```python
from build123d import *

# Parameters (mm, degrees)
F0_W     = 50
F0_H     = 7
F1_DEPTH = 25
F2_SIZE  = 2.4
F3_R     = 0.6
F4_DEPTH = 16.5
F5_R     = 0.59999


# Not quite as in the source:
# - a fillet or chamfer is up to 0.001 mm smaller than in the source, because OpenCascade refuses the exact size


with BuildPart() as f1:
    # F0 (on Top) → F1 (new body)
    with BuildSketch(Plane.XY):
        Rectangle(F0_W, F0_H)
    extrude(amount=F1_DEPTH)

    # F2
    f2_edges = [f1.edges().sort_by_distance(p)[0] for p in [
        (0, -3.5, 25),
        (0, 3.5, 25),
    ]]
    chamfer(f2_edges, length=F2_SIZE)

    # F3 (on Right) → F4 (join, symmetric)
    with BuildSketch(Plane.YZ):
        with Locations((0, 25)):
            Circle(F3_R)
    extrude(amount=F4_DEPTH, both=True)

    # F5 (radius 0.6 in the source; OpenCascade refuses exactly that, so slightly less here)
    f5_edges = [f1.edges().sort_by_distance(p)[0] for p in [
        (16.5, 0, 25.6),
        (-16.5, 0, 25.6),
    ]]
    fillet(f5_edges, radius=F5_R)


solid = f1.part
```
CAD build for the part. Positions are in the model's coordinates, mm. A direction names the side the tool comes from. Round coordinates to 2 decimals unless told otherwise and drop trailing zeros. Order: outer loops, then holes, each group sorted by start corner. A loop starts at its lowest first (then second) coordinate and runs counter-clockwise, first axis right, second up.
Item 1: Saw through at B-B on y = 2.5. Write the cut outline in (x, z).
Item 2: Pin check, flat tips, straight feed: pin 1 (0.7 mm diameter, centred on x = -5.5, y = 0.5, fed in from +Z); pin 2 (3 mm diameter, centred on x = -19.5, y = 2.5, fed in from +Z). Stop position of each tip, or through.
Item 3: Tool access for faces 1 (the face through (0.2, 0, 25.6)), 2 (the face through (-0.35, 0.75, 25)): list every direction of +Z, -Z, +X, -X, +Y, -Y with a clear straight run to the whole face (end or side of a thin tool).
Item 4: Saw through at A-A on x = -21. Write the cut outline in (y, z).
Item 5: Probe line 1 along Z through (x, y) = (-18.5, 1); line 2 along Z through (x, y) = (-16, 0); line 3 along Y through (x, z) = (-4, 23). List the from-to ranges inside material, lowest first.
Item 6: Saw through at C-C on x = 9.5. Write the cut outline in (y, z).
Reported:
1. outline: (-25, 0) - (25, 0) - (25, 23.6) - (-25, 23.6) - close
2. pin 1: stops at z = 25.58
2. pin 2: stops at z = 25
3. face 1: +Z, +X, -X
3. face 2: +Z
4. outline: (-3.5, 0) - (3.5, 0) - (3.5, 22.6) - (1.1, 25) - (-1.1, 25) - (-3.5, 22.6) - close
5. line 1: z = 0 to 25
5. line 2: z = 0 to 25.59
5. line 3: y = -3.1 to 3.1
6. outline: (-3.5, 0) - (3.5, 0) - (3.5, 22.6) - (1.1, 25) - (0.6, 25) arc R0.6 ccw to (-0.6, 25) - (-1.1, 25) - (-3.5, 22.6) - close
